The listing builds one solid part. Answer for the finished solid, in the listing's coordinates (mm). A direction names the side the tool comes from. Round coordinates to 2 decimals unless told otherwise and drop trailing zeros. Order: outer loops, then holes, each group sorted by start corner. A loop starts at its lowest first (then second) coordinate and runs counter-clockwise, first axis right, second up. Notation, with made-up numbers: (31.5, -17.5) -> (73.5, -17.5) arc R10 cw to (73.5, -12.5) -> close; hole circle Ø9 at (54, 48.5). An arc over 180 degrees is marked (long way). Answer in a Markdown table with one row per item. Add a question column.
```python
from build123d import *

# Parameters (mm, degrees)
SKETCH3_W           = 60
SKETCH3_H           = 80
BOSS_EXTRUDE1_DEPTH = 25
SKETCH4_W           = 60
SKETCH4_H           = 80
BOSS_EXTRUDE2_DEPTH = 25
BOSS_EXTRUDE3_DEPTH = 240
BOSS_EXTRUDE4_DEPTH = 240


with BuildPart() as part:
    # Sketch3 → Boss-Extrude1 (new body)
    with BuildSketch(Plane(origin=(0, -266.5409196, 0), x_dir=(-1, 0, 0), z_dir=(0, -1, 0))):
        with Locations((-150, 40)):
            Rectangle(SKETCH3_W, SKETCH3_H)
    extrude(amount=BOSS_EXTRUDE1_DEPTH)



with BuildPart() as body_2:
    # Sketch4 → Boss-Extrude2 (new body)
    with BuildSketch(Plane(origin=(0, -26.5409196, 0), x_dir=(1, 0, 0), z_dir=(0, 1, 0))):
        with Locations((150, 40)):
            Rectangle(SKETCH4_W, SKETCH4_H)
    extrude(amount=BOSS_EXTRUDE2_DEPTH)


with BuildPart() as part_1:
    add(part.part)

    add(body_2.part)  # Boss-Extrude3 merges body 2
    # Sketch5 → Boss-Extrude3 (add)
    with BuildSketch(Plane(origin=(0, -266.5409196, 0), x_dir=(1, 0, 0), z_dir=(0, 1, 0))):
        Polygon((120, 80), (180, 0), (120, 0), align=None)
    extrude(amount=BOSS_EXTRUDE3_DEPTH)

    # Sketch6 → Boss-Extrude4 (add)
    with BuildSketch(Plane(origin=(0, -266.5409196, 0), x_dir=(1, 0, 0), z_dir=(0, 1, 0))):
        Polygon((120, 80), (180, 80), (120, 0), align=None)
    extrude(amount=BOSS_EXTRUDE4_DEPTH)


solid = part_1.part
```
1. The part is cut by section A-A (z = -62). Give the vertices of the cut face in (x, y), then the cut area to 3 significant figures.
2. The part is cut by section B-B (y = -203). Give the vertices of the cut face in (x, z).
3. Straight lines are drawn through the part: line 1 along Y through (x, z) = (164, -42.5); line 2 along Z through (x, y) = (150.5, -40.5); line 3 along Z through (x, y) = (177, -253). For each, find the intervals that lie inside material, in ascending order.
4. The part is cut by section D-D (z = -30). Give the vertices of the cut face in (x, y), then the cut area to 3 significant figures.
5. For faces 1 (the flat face through (180, -14, -39)), 2 (the flat face through (169, -266.541, -41)), determine the directions among +Z, -Z, +X, -X, +Y, -Y from which every point of the face is accessible in a straight line to the end or side of a thin tool.
6. The part is cut by section C-C (x = 171.5). Give the vertices of the cut face in (y, z), then the cut area to 3 significant figures.
7. The mould has two halves that part along Z. Classify faces 3 (the flat face through (168, -26.541, -41)), 4 (the flat face through (150, -149, 0)), 5 (the flat face through (150, -149, -80)): released by +Z, released by -Z, zero draft, split by the parting line, or undercut.
Report:
| question | item | result |
|---|---|---|
| 1 | outline | (120, -291.54) -> (180, -291.54) -> (180, -266.54) -> (166.5, -266.54) -> (166.5, -26.54) -> (180, -26.54) -> (180, -1.54) -> (120, -1.54) -> close |
| 1 | area | 14,200 mm^2 |
| 2 | outline | (120, -80) -> (180, -80) -> (150, -40) -> (180, 0) -> (120, 0) -> close |
| 3 | line 1 | y = -291.54 to -266.54, -26.54 to -1.54 |
| 3 | line 2 | z = -80 to -40.67, -39.33 to 0 |
| 3 | line 3 | z = -80 to -76, -4 to 0 |
| 4 | outline | (120, -291.54) -> (180, -291.54) -> (180, -266.54) -> (157.5, -266.54) -> (157.5, -26.54) -> (180, -26.54) -> (180, -1.54) -> (120, -1.54) -> close |
| 4 | area | 12,000 mm^2 |
| 5 | face 1 | +Z, -Z, +X, +Y, -Y |
| 5 | face 2 | +X |
| 6 | outline | (-291.54, -80) -> (-1.54, -80) -> (-1.54, 0) -> (-291.54, 0) -> close; hole (-266.54, -68.67) -> (-26.54, -68.67) -> (-26.54, -11.33) -> (-266.54, -11.33) -> close |
| 6 | area | 9,440 mm^2 |
| 7 | face 3 | undercut |
| 7 | face 4 | released by +Z |
| 7 | face 5 | released by -Z |
